Read the model definition and answer for the solid it produces. Units are mm, in the model's axes. Give positions to 0.01 mm unless a question says otherwise; leave off trailing zeros. Order: outer loops, then holes, each group sorted by start corner. A loop starts at its lowest first (then second) coordinate and runs counter-clockwise, first axis right, second up. Notation, with made-up numbers: (-36, 16.25) - (-13, 16.25) arc R17 ccw to (-13, 43.25) - close; hole circle Ø9 at (-5, -4). An arc over 180 degrees is marked (long way). Answer as CSV lines item,"result". Start each with the question number.
Autodesk Inventor part; units mm, degrees
ref_plane "Work Plane1" through (32, 0, 0) normal (1, 0, 0) x (0, 1, 0)
ref_plane "XZ Plane" through (0, 0, 0) normal (0, 1, 0) x (-1, 0, 0)
ref_plane "XY Plane" through (0, 0, 0) normal (0, 0, 1) x (1, 0, 0)
sketch "Sketch1" plane through (0, 0, 0) normal (0, 1, 0) x (-1, 0, 0)
  circle A0 centre (0, 0) radius 32
  dimension "d0" = 64
extrude "Extrusion1" add sketch "Sketch1" along normal blind 10
sketch "Sketch2" plane through (0, 10, 0) normal (0, 1, 0) x (1, 0, 0)
  circle A0 centre (0, 0) radius 30.5
  dimension "d3" = 61
extrude "Extrusion2" cut sketch "Sketch2" against normal blind 8
ref_plane "Work Plane1" through (32, 0, 0) normal (1, 0, 0) x (0, 1, 0)
sketch "Sketch5" plane through (32, 0, 0) normal (1, 0, 0) x (0, 1, 0)
  circle A0 centre (5, 0) radius 1.5
  line L0 (10, -32) -> (10, 32)
  point P0 (0, 0)
  dimension "d7" = 3
  dimension "d8" = 5
extrude "Extrusion3" cut sketch "Sketch5" against normal through all
properties part number "bouchon"
(1) Section B-B, the plane x = 0 is taken. Write down the section's boundary in (y, z).
(2) Flat-ended cylindrical pins translate along their axes: pin 1 Ø1.5 at (x, z) = (-23, -16.5) entering from +Y; pin 2 Ø4 at (y, z) = (2, -15.5) entering from +X; pin 3 Ø5 at (x, z) = (13, -7.5) entering from -Y; pin 4 Ø2.5 at (y, z) = (5, 0) entering from +X. Find the tip coordinate at first contact, or state that the pin passes through.
(3) Determine the mould class of faces 1 (the flat face through (0, 0, 0)), 2 (the cylindrical face through (28.174, 6.056, 11.682)), 3 (the flat face through (0, 2, 0)), 4 (the cylindrical face through (-29.56, 4.93, 12.26)) for opening direction X: released by +X, released by -X, zero draft, split by the parting line, or undercut.
(4) Section A-A, the plane z = 0 is taken. Write down the section's boundary in (x, y).
(5) Straight lines are drawn through the part: line 1 (Y direction, x = -31.45, z = 0); line 2 (Z direction, x = 0, y = 8); line 3 (Y direction, x = 22.5, z = -3.5). For each, find the intervals that lie inside material, in ascending order. Write a range as [from, to].
(6) Section D-D, the plane y = 8.75 is taken. Write down the section's boundary in (x, z), and give its area (3 significant figures).
Checks:
1,outline,"(0, -32) - (10, -32) - (10, -30.5) - (2, -30.5) - (2, 30.5) - (10, 30.5) - (10, 32) - (0, 32) - close"
2,pin 1,"stops at y = 2"
2,pin 2,"stops at x = 29.01"
2,pin 3,"stops at y = 0"
2,pin 4,"passes through"
3,face 1,"zero draft"
3,face 2,"undercut"
3,face 3,"undercut"
3,face 4,"split by the parting line"
4,outline,"(-32, 0) - (32, 0) - (32, 3.5) - (30.5, 3.5) - (30.5, 2) - (-30.5, 2) - (-30.5, 3.5) - (-32, 3.5) - close; (-32, 6.5) - (-30.5, 6.5) - (-30.5, 10) - (-32, 10) - close; (30.5, 6.5) - (32, 6.5) - (32, 10) - (30.5, 10) - close"
5,line 1,"y = [0, 3.5], [6.5, 10]"
5,line 2,"z = [-32, -30.5], [30.5, 32]"
5,line 3,"y = [0, 2]"
6,outline,"circle Ø64 at (0, 0); hole circle Ø61 at (0, 0)"
6,area,"295 mm²"
